The model under review builds one solid part; all positions refer to its coordinate system, in mm. A direction names the side the tool comes from. Coordinates: 2 decimals unless noted, no trailing zeros. Order: outer loops, then holes, each group sorted by start corner. A loop starts at its lowest first (then second) coordinate and runs counter-clockwise, first axis right, second up. Notation, with made-up numbers: (-39, 35) -> (-1, 35) arc R20 cw to (-1, 63) -> close; hole circle Ø2 at (55, -17). An arc over 180 degrees is marked (long way). Put each result on its own line as item: value.
Autodesk Inventor part; units mm, degrees
ref_plane "YZ Plane" through (0, 0, 0) normal (1, 0, 0) x (0, 1, 0)
ref_plane "XZ Plane" through (0, 0, 0) normal (0, 1, 0) x (-1, 0, 0)
ref_plane "XY Plane" through (0, 0, 0) normal (0, 0, 1) x (1, 0, 0)
sketch "Sketch1" plane through (0, 0, 0) normal (0, 1, 0) x (-1, 0, 0)
  circle A0 centre (0, 0) radius 15
  dimension "d0" = 30
sketch "Sketch2" plane through (0, 0, 0) normal (0, 1, 0) x (-1, 0, 0)
  line L0 (0, 0) -> (22.5, 0)
  line L1 (0, 0) -> (-22.5, 0)
  line L2 (-22.5, 0) -> (-22.5, -20)
  line L3 (-22.5, 0) -> (-22.5, 20)
  line L4 (22.5, 0) -> (22.5, -20)
  line L5 (22.5, -20) -> (-22.5, -20)
  line L6 (22.5, 0) -> (22.5, 20)
  line L7 (22.5, 20) -> (-22.5, 20)
  dimension "d1" = 22.5
  dimension "d2" = 22.5
  dimension "d3" = 20
  dimension "d4" = 20
sketch "Sketch3" plane through (0, 0, 0) normal (0, 1, 0) x (-1, 0, 0)
  circle A0 centre (0, 0) radius 7.5
  dimension "d5" = 15
extrude "Extrusion1" add sketch "Sketch1" along normal mid plane 66
extrude "Extrusion2" add sketch "Sketch2" along normal mid plane 45
extrude "Extrusion3" cut sketch "Sketch3" along normal mid plane 100
sketch "Sketch4" plane through (-22.5, 22.5, 20) normal (0, 0, 1) x (1, 0, 0)
  line L0 (10.5, -22.5) -> (10.5, -37.5)
  line L1 (10.5, -37.5) -> (34.5, -37.5)
  line L2 (34.5, -37.5) -> (34.5, -22.5)
  line L3 (10.5, -22.5) -> (10.5, -7.5)
  line L4 (10.5, -7.5) -> (34.5, -7.5)
  line L5 (34.5, -7.5) -> (34.5, -22.5)
  point P0 (22.5, -22.5)
  dimension "d14" = 15
sketch "Sketch5" plane through (22.5, -22.5, -20) normal (1, 0, 0) x (0, 0, -1)
  circle A0 centre (-20, 22.5) radius 17.5
  dimension "d15" = 35
sketch "Sketch6" plane through (22.5, -22.5, -20) normal (1, 0, 0) x (0, 0, -1)
  circle A0 centre (-20, 22.5) radius 9
  dimension "d28" = 18
extrude "Extrusion4" add sketch "Sketch5" along normal blind 22
sketch "Sketch7" plane through (-22.5, -22.5, 20) normal (-1, 0, 0) x (0, 0, 1)
  circle A0 centre (-20, 22.5) radius 17.5
  dimension "d20" = 35
extrude "Extrusion5" add sketch "Sketch7" along normal blind 22
extrude "Extrusion6" cut sketch "Sketch4" against normal blind 100
extrude "Extrusion7" cut sketch "Sketch6" along normal mid plane 200
properties part number "Sólido 1"
Item 1: For line 1 (Y direction, x = 2, z = -10.5); line 2 (Y direction, x = -36, z = 0); line 3 (Z direction, x = 0, y = -18.5), list the stretches that pass through material, from the lowest coordinate up. Write a range as from..to.
Answers below:
line 1: -33..-15, 15..33
line 2: -17.5..-9, 9..17.5
line 3: -20..-7.5, 7.5..20
Item 2: Consider section A-A on x = 0. Write out the cut boundary in (y, z).
Answers below:
outline: (-33, -15) -> (-22.5, -15) -> (-22.5, -20) -> (-15, -20) -> (-15, -7.5) -> (-33, -7.5) -> close; (-33, 7.5) -> (-15, 7.5) -> (-15, 20) -> (-22.5, 20) -> (-22.5, 15) -> (-33, 15) -> close; (15, -20) -> (22.5, -20) -> (22.5, -15) -> (33, -15) -> (33, -7.5) -> (15, -7.5) -> close; (15, 7.5) -> (33, 7.5) -> (33, 15) -> (22.5, 15) -> (22.5, 20) -> (15, 20) -> close
Item 3: Consider section C-C on z = 0. Count the separate pieces of the cut face and the enclosed holes in it, and give its area (4 significant figures).
Answers below:
separate pieces: 4
enclosed holes: 0
area: 1,765 mm^2
Item 4: Consider section B-B on y = 0. Write out the cut boundary in (x, z).
Answers below:
outline: (-44.5, -17.5) -> (-22.5, -17.5) -> (-22.5, -20) -> (-12, -20) -> (-12, -9) -> (-44.5, -9) -> close; (-44.5, 9) -> (-12, 9) -> (-12, 20) -> (-22.5, 20) -> (-22.5, 17.5) -> (-44.5, 17.5) -> close; (12, -20) -> (22.5, -20) -> (22.5, -17.5) -> (44.5, -17.5) -> (44.5, -9) -> (12, -9) -> close; (12, 9) -> (44.5, 9) -> (44.5, 17.5) -> (22.5, 17.5) -> (22.5, 20) -> (12, 20) -> close
Item 5: Mouldability with a two-part tool opening along Y and no side actions: class faces 6 (the flat face through (-8, 15, 0)), 7 (the cylindrical face through (14.985, -27.676, 0.66)), 8 (the cylindrical face through (33.346, 10.648, 13.887)) as +Y half, -Y half, draft (parallel to the pull), parting line (faces both ways), or undercut.
Answers below:
face 6: undercut
face 7: draft
face 8: parting line
Item 6: Consider section D-D on y = 16.5. Write out the cut boundary in (x, z).
Answers below:
outline: (-44.5, -5.83) -> (-22.5, -5.83) -> (-22.5, -20) -> (22.5, -20) -> (22.5, -5.83) -> (44.5, -5.83) -> (44.5, 5.83) -> (22.5, 5.83) -> (22.5, 20) -> (-22.5, 20) -> (-22.5, 5.83) -> (-44.5, 5.83) -> close; hole circle Ø15 at (0, 0)
Item 7: For faces 1 (the cylindrical face through (-33.346, 10.648, -13.887)), 2 (the cylindrical face through (14.985, 27.676, -0.66)), 3 (the flat face through (-0.3, -15.3, -20)), 4 (the flat face through (-8, -15, 0)), 5 (the flat face through (22.5, -15.3, -9.2)), list the 3-axis set-ups (+Z, -Z, +X, -X, +Y, -Y) from which the entire face can be reached by the end or side of a thin tool; tool diameter is ignored.
Answers below:
face 1: -X
face 2: +Y
face 3: -Z, +X, -X, +Y, -Y
face 4: +Z, -Z
face 5: +X
Item 8: For pin 1 Ø4 at (y, z) = (17, -14) entering from -X; pin 2 Ø1.5 at (x, z) = (-24, 8) entering from +Y; pin 3 Ø8 at (y, z) = (-25, 14) entering from +X, all flat-tipped, find the tip position at first contact; note any pin that passes through.
Answers below:
pin 1: x = -22.5
pin 2: y = 15.93
pin 3: x = 22.5
